The listing builds one solid part. Answer for the finished solid, in the listing's coordinates (mm). Coordinates: 2 decimals unless noted, no trailing zeros. Order: outer loops, then holes, each group sorted by start corner. A loop starts at its lowest first (then second) coordinate and runs counter-clockwise, first axis right, second up. Notation, with made-up numbers: (-23, 76.5) -> (6, 76.5) arc R26 cw to (6, 111.5) -> close; hole circle Ø4 at (33, 31.25). An arc over 180 degrees is marked (long way). Put each result on its own line as item: value. Start each with the question number.
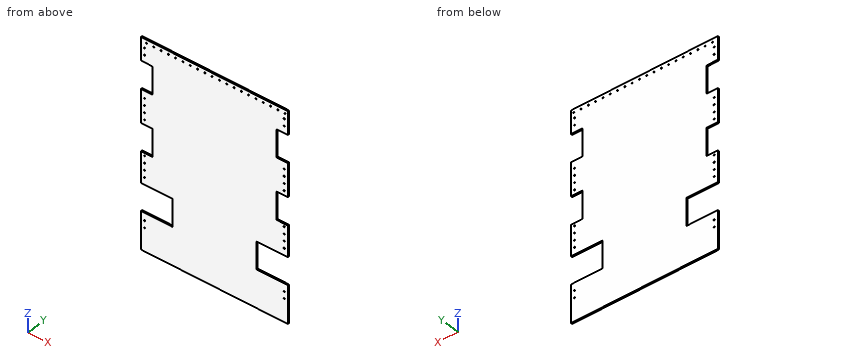
```python
from build123d import *

# Parameters (mm, degrees)
CROQUIS1_W              = 511
CROQUIS1_H              = 705.8
SALIENTE_EXTRUIR1_DEPTH = 5
CROQUIS2_W              = 40
CROQUIS2_H              = 100
CORTAR_EXTRUIR1_DEPTH   = 10
CROQUIS4_W              = 110
CROQUIS4_H              = 98.950839499
CORTAR_EXTRUIR3_DEPTH   = 10
CROQUIS7_R              = 2.07
CORTAR_EXTRUIR6_DEPTH   = 10
CROQUIS8_R              = 2.07
CORTAR_EXTRUIR7_DEPTH   = 10
CROQUIS9_W              = 511
CROQUIS9_H              = 45
SALIENTE_EXTRUIR2_DEPTH = 5


with BuildPart() as part:
    # Croquis1 → Saliente-Extruir1 (new body)
    with BuildSketch(Plane(origin=(0, 0, 0), x_dir=(1, 0, 0), z_dir=(0, 1, 0))):
        Rectangle(CROQUIS1_W, CROQUIS1_H)
    extrude(amount=SALIENTE_EXTRUIR1_DEPTH)

    # Croquis2 → Cortar-Extruir1 (cut)
    with BuildSketch(Plane(origin=(0, 0, 0), x_dir=(-1, 0, 0), z_dir=(0, -1, 0))):
        with Locations((235.5, -219.401276077)):
            Rectangle(CROQUIS2_W, CROQUIS2_H)
        with Locations((-235.5, -219.401276077)):
            Rectangle(CROQUIS2_W, CROQUIS2_H)
        with Locations((235.5, 0.598723923)):
            Rectangle(CROQUIS2_W, CROQUIS2_H)
        with Locations((-235.5, 0.598723923)):
            Rectangle(CROQUIS2_W, CROQUIS2_H)
    extrude(amount=-CORTAR_EXTRUIR1_DEPTH, mode=Mode.SUBTRACT)

    # Croquis4 → Cortar-Extruir3 (cut)
    with BuildSketch(Plane(origin=(0, 0, 0), x_dir=(-1, 0, 0), z_dir=(0, -1, 0))):
        with Locations((200.5, 211.875419749)):
            Rectangle(CROQUIS4_W, CROQUIS4_H)
        with Locations((-200.9, 211.875419749)):
            Rectangle(CROQUIS4_W, CROQUIS4_H)
    extrude(amount=-CORTAR_EXTRUIR3_DEPTH, mode=Mode.SUBTRACT)

    # Croquis7 → Cortar-Extruir6 (cut)
    with BuildSketch(Plane(origin=(0, 0, 0), x_dir=(-1, 0, 0), z_dir=(0, -1, 0))):
        with Locations(Location((236.6, -340.2, 0), (0, 0, 90))):
            Circle(CROQUIS7_R)
        with Locations(Location((211.2, -340.2, 0), (0, 0, 90))):
            Circle(CROQUIS7_R)
        with Locations(Location((185.8, -340.2, 0), (0, 0, 90))):
            Circle(CROQUIS7_R)
        with Locations(Location((160.4, -340.2, 0), (0, 0, 90))):
            Circle(CROQUIS7_R)
        with Locations(Location((135, -340.2, 0), (0, 0, 90))):
            Circle(CROQUIS7_R)
        with Locations(Location((109.6, -340.2, 0), (0, 0, 90))):
            Circle(CROQUIS7_R)
        with Locations(Location((84.2, -340.2, 0), (0, 0, 90))):
            Circle(CROQUIS7_R)
        with Locations(Location((58.8, -340.2, 0), (0, 0, 90))):
            Circle(CROQUIS7_R)
        with Locations(Location((33.4, -340.2, 0), (0, 0, 90))):
            Circle(CROQUIS7_R)
        with Locations(Location((8, -340.2, 0), (0, 0, 90))):
            Circle(CROQUIS7_R)
        with Locations(Location((-17.4, -340.2, 0), (0, 0, 90))):
            Circle(CROQUIS7_R)
        with Locations(Location((-42.8, -340.2, 0), (0, 0, 90))):
            Circle(CROQUIS7_R)
        with Locations(Location((-68.2, -340.2, 0), (0, 0, 90))):
            Circle(CROQUIS7_R)
        with Locations(Location((-93.6, -340.2, 0), (0, 0, 90))):
            Circle(CROQUIS7_R)
        with Locations(Location((-119, -340.2, 0), (0, 0, 90))):
            Circle(CROQUIS7_R)
        with Locations(Location((-144.4, -340.2, 0), (0, 0, 90))):
            Circle(CROQUIS7_R)
        with Locations(Location((-169.8, -340.2, 0), (0, 0, 90))):
            Circle(CROQUIS7_R)
        with Locations(Location((-195.2, -340.2, 0), (0, 0, 90))):
            Circle(CROQUIS7_R)
        with Locations(Location((-220.6, -340.2, 0), (0, 0, 90))):
            Circle(CROQUIS7_R)
        with Locations(Location((-246, -340.2, 0), (0, 0, 90))):
            Circle(CROQUIS7_R)
        with Locations(Location((242.8, -320.2, 0), (0, 0, 90))):
            Circle(CROQUIS7_R)
        with Locations(Location((242.8, -294.8, 0), (0, 0, 90))):
            Circle(CROQUIS7_R)
        with Locations(Location((242.8, -142.4, 0), (0, 0, 90))):
            Circle(CROQUIS7_R)
        with Locations(Location((242.8, -117, 0), (0, 0, 90))):
            Circle(CROQUIS7_R)
        with Locations(Location((242.8, -91.6, 0), (0, 0, 90))):
            Circle(CROQUIS7_R)
        with Locations(Location((242.8, -66.2, 0), (0, 0, 90))):
            Circle(CROQUIS7_R)
        with Locations(Location((242.8, 60.8, 0), (0, 0, 90))):
            Circle(CROQUIS7_R)
        with Locations(Location((242.8, 86.2, 0), (0, 0, 90))):
            Circle(CROQUIS7_R)
        with Locations(Location((242.8, 111.6, 0), (0, 0, 90))):
            Circle(CROQUIS7_R)
        with Locations(Location((242.8, 137, 0), (0, 0, 90))):
            Circle(CROQUIS7_R)
        with Locations(Location((242.8, 289.4, 0), (0, 0, 90))):
            Circle(CROQUIS7_R)
        with Locations(Location((242.8, 314.8, 0), (0, 0, 90))):
            Circle(CROQUIS7_R)
    extrude(amount=-CORTAR_EXTRUIR6_DEPTH, mode=Mode.SUBTRACT)

    # Croquis8 → Cortar-Extruir7 (cut)
    with BuildSketch(Plane(origin=(0, 0, 0), x_dir=(-1, 0, 0), z_dir=(0, -1, 0))):
        with Locations((246, 385.2)):
            Circle(CROQUIS8_R)
        with Locations((220.6, 385.2)):
            Circle(CROQUIS8_R)
        with Locations((195.2, 385.2)):
            Circle(CROQUIS8_R)
        with Locations((169.8, 385.2)):
            Circle(CROQUIS8_R)
        with Locations((144.4, 385.2)):
            Circle(CROQUIS8_R)
        with Locations((119, 385.2)):
            Circle(CROQUIS8_R)
        with Locations((93.6, 385.2)):
            Circle(CROQUIS8_R)
        with Locations((68.2, 385.2)):
            Circle(CROQUIS8_R)
        with Locations((42.8, 385.2)):
            Circle(CROQUIS8_R)
        with Locations((17.4, 385.2)):
            Circle(CROQUIS8_R)
        with Locations((-8, 385.2)):
            Circle(CROQUIS8_R)
        with Locations((-33.4, 385.2)):
            Circle(CROQUIS8_R)
        with Locations((-58.8, 385.2)):
            Circle(CROQUIS8_R)
        with Locations((-84.2, 385.2)):
            Circle(CROQUIS8_R)
        with Locations((-109.6, 385.2)):
            Circle(CROQUIS8_R)
        with Locations((-135, 385.2)):
            Circle(CROQUIS8_R)
        with Locations((-160.4, 385.2)):
            Circle(CROQUIS8_R)
        with Locations((-185.8, 385.2)):
            Circle(CROQUIS8_R)
        with Locations((-211.2, 385.2)):
            Circle(CROQUIS8_R)
        with Locations((-236.6, 385.2)):
            Circle(CROQUIS8_R)
        with Locations(Location((-242.8, 314.8, 0), (0, 0, 90))):
            Circle(CROQUIS8_R)
        with Locations(Location((-242.8, 289.4, 0), (0, 0, 90))):
            Circle(CROQUIS8_R)
        with Locations(Location((-242.8, 137, 0), (0, 0, 90))):
            Circle(CROQUIS8_R)
        with Locations(Location((-242.8, 111.6, 0), (0, 0, 90))):
            Circle(CROQUIS8_R)
        with Locations(Location((-242.8, 86.2, 0), (0, 0, 90))):
            Circle(CROQUIS8_R)
        with Locations(Location((-242.8, 60.8, 0), (0, 0, 90))):
            Circle(CROQUIS8_R)
        with Locations(Location((-242.8, -66.2, 0), (0, 0, 90))):
            Circle(CROQUIS8_R)
        with Locations(Location((-242.8, -91.6, 0), (0, 0, 90))):
            Circle(CROQUIS8_R)
        with Locations(Location((-242.8, -117, 0), (0, 0, 90))):
            Circle(CROQUIS8_R)
        with Locations(Location((-242.8, -142.4, 0), (0, 0, 90))):
            Circle(CROQUIS8_R)
        with Locations(Location((-242.8, -294.8, 0), (0, 0, 90))):
            Circle(CROQUIS8_R)
        with Locations(Location((-242.8, -320.2, 0), (0, 0, 90))):
            Circle(CROQUIS8_R)
    extrude(amount=-CORTAR_EXTRUIR7_DEPTH, mode=Mode.SUBTRACT)

    # Croquis9 → Saliente-Extruir2 (add)
    with BuildSketch(Plane(origin=(0, 5, 0), x_dir=(1, 0, 0), z_dir=(0, 1, 0))):
        with Locations((0, 375.4)):
            Rectangle(CROQUIS9_W, CROQUIS9_H)
    extrude(amount=-SALIENTE_EXTRUIR2_DEPTH)


solid = part.part
```
(1) Each of these flat-tipped pins is pushed along its axis until it touches: P1, Ø2, axis at y = 2.5, z = 246, coming from the -X side; P2, Ø5, axis at x = -160.4, z = 340.2, coming from the -Y side. Where does it stop, or does it pass through?
(2) The part is cut by section C-C on z = -208.5. Determine the outline of the cut face in (x, y), plus the area to 3 significant figures.
(3) The part is cut by section B-B on y = 1.65. Count the separate pieces of the cut face and the enclosed holes in it, plus the area to 3 significant figures.
(4) The part is cut by section A-A on z = 191. Determine the outline of the cut face in (x, y).
(5) Find the intervals of material crossed by L1, parallel to Z at x = -185, y = 1.75; L2, parallel to X at y = 2.5, z = 91.6; L3, parallel to Z at x = 68.5, y = 1.2, in increasing order.
Worked out:
1. P1: x = -215.5
1. P2: y = 0
2. outline: (-145.5, 0) -> (145.9, 0) -> (145.9, 5) -> (-145.5, 5) -> close
2. area: 1,460 mm2
3. separate pieces: 1
3. enclosed holes: 44
3. area: 345,000 mm2
4. outline: (-215.5, 0) -> (215.5, 0) -> (215.5, 5) -> (-215.5, 5) -> close
5. L1: -397.9 to -261.35, -162.4 to 338.29, 342.11 to 352.9
5. L2: -255.5 to -244.87, -240.73 to 240.73, 244.87 to 255.5
5. L3: -397.9 to 338.15, 342.25 to 352.9
